from build123d import *

# Parameters (mm, degrees)
F0_W     = 40.64
F0_H     = 20.32
F1_DEPTH = 4.1275
F2_W     = 25.4
F2_H     = 12.7
F3_DEPTH = 1.905


with BuildPart() as f1:
    # F0 (on Top) → F1 (new body, symmetric)
    with BuildSketch(Plane.XY):
        Rectangle(F0_W, F0_H)
    extrude(amount=F1_DEPTH, both=True)

    # F2 (on Top) → F3 (cut, symmetric)
    with BuildSketch(Plane.XY):
        Rectangle(F2_W, F2_H)
    extrude(amount=F3_DEPTH, both=True, mode=Mode.SUBTRACT)


solid = f1.part
For this review, take the finished solid that the model builds, in its own axes (mm). A direction names the side the tool comes from. Round coordinates to 2 decimals unless told otherwise and drop trailing zeros. Loops run counter-clockwise (first coordinate to the right, second up) from the corner with the lowest first, then second, coordinate; pieces in that order, holes last. Notation, with made-up numbers: (-40, 44) - (-6, 44) arc R26 cw to (-6, 58) - close; hole circle Ø11 at (67, 37). An arc over 180 degrees is marked (long way). One line per item, written item: value. Start each with the question number.
Item 1: The part is to be moulded in two halves that separate along Z. For faces 1 (the flat face through (0, 0, -4.128)), 2 (the flat face through (0, 0, 4.128)), 3 (the flat face through (0, 10.16, 0)), 4 (the flat face through (0, 0, -1.905)), say which applies: +Z half, -Z half, draft (parallel to the pull), parting line (faces both ways), or undercut.
Item 2: For L1, parallel to Z at x = -4.5, y = 3.5 (1 decimal); L2, parallel to Y at x = -11, z = -1.5; L3, parallel to X at y = -1, z = 0.5, list the stretches that pass through material, from the lowest coordinate up.
Item 3: For faces 5 (the flat face through (20.32, 0, 0)), 6 (the flat face through (0, 0, 1.905)), list the 3-axis set-ups (+Z, -Z, +X, -X, +Y, -Y) from which the entire face can be reached by the end or side of a thin tool; tool diameter is ignored.
Item 4: Take a section at A-A (z = -1.25). Give the boundary of the cut face in (x, y), plus the area to 3 significant figures.
Answer below:
1. face 1: -Z half
1. face 2: +Z half
1. face 3: draft
1. face 4: undercut
2. L1: z = -4.1 to -1.9, 1.9 to 4.1
2. L2: y = -10.16 to -6.35, 6.35 to 10.16
2. L3: x = -20.32 to -12.7, 12.7 to 20.32
3. face 5: +Z, -Z, +X, +Y, -Y
3. face 6: none
4. outline: (-20.32, -10.16) - (20.32, -10.16) - (20.32, 10.16) - (-20.32, 10.16) - close; hole (-12.7, -6.35) - (12.7, -6.35) - (12.7, 6.35) - (-12.7, 6.35) - close
4. area: 503 mm2
